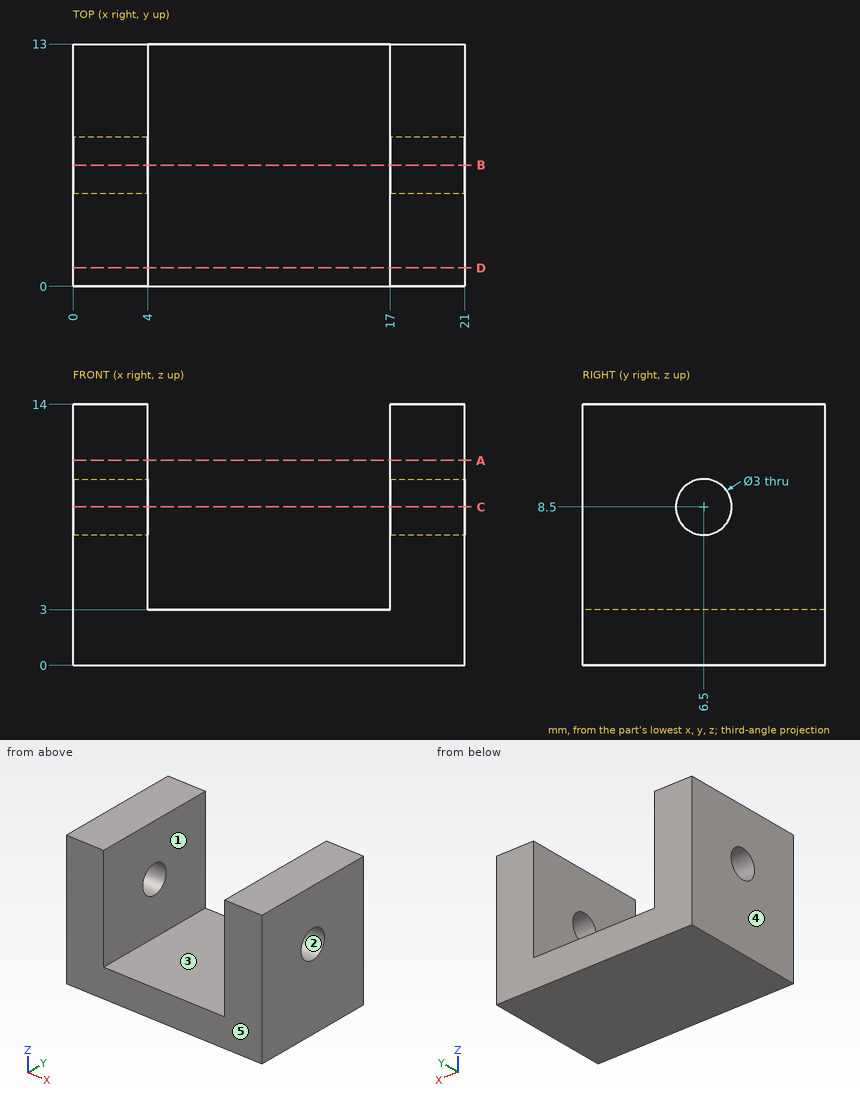
The figure shows three views and two pictorial views of one solid part (mm, origin at its lowest corner). Answer the questions. A direction names the side the tool comes from. Round coordinates to 2 decimals unless told otherwise and drop trailing zeros. Write each loop counter-clockwise with the first axis right and the second up, starting at its lowest first coordinate (ties: lowest second). Pieces come first, ordered by that corner, then holes. Notation, with made-up numbers: (-37.5, 5.25) - (-6.5, 5.25) arc R19 ccw to (-6.5, 11.25) - close; hole circle Ø10 at (85.25, -13.75). An arc over 180 degrees is marked (long way). Use one line per item in the form item = value. Start each with the question number.
Item 1: A cutting plane is placed at A-A (z = 11). Write down the section's boundary in (x, y), plus the area to 3 significant figures.
Item 2: A cutting plane is placed at D-D (y = 1). Write down the section's boundary in (x, z).
Item 3: Determine the mould class of the marked faces 3, 4 and 5 for opening direction X: +X half, -X half, draft (parallel to the pull), parting line (faces both ways), or undercut.
Item 4: A cutting plane is placed at B-B (y = 6.5). Write down the section's boundary in (x, z).
Item 5: Find the intervals of material crossed by line 1 (X direction, y = 3.75, z = 11); line 2 (Z direction, x = 19.9, y = 6.5); line 3 (Z direction, x = 12.5, y = 10.5), in increasing order. Write a range as [from, to].
Item 6: Flat-ended cylindrical pins translate along their axes: pin 1 Ø1.5 at (x, y) = (11, 10.5) entering from +Z; pin 2 Ø4 at (x, z) = (14, 6) entering from -Y. Find the tip coordinate at first contact, or state that the pin passes through.
Item 7: A cutting plane is placed at C-C (z = 8.5). Write down the section's boundary in (x, y).
Item 8: A tool of negligible diameter and unlimited length cuts with its end or side. For the marked faces 1 and 2, from which of +Z, -Z, +X, -X, +Y, -Y can it reach the whole face along a straight path? Write none if from no direction.
The answers:
q1.outline = (0, 0) - (4, 0) - (4, 13) - (0, 13) - close; (17, 0) - (21, 0) - (21, 13) - (17, 13) - close
q1.area = 104 mm^2
q2.outline = (0, 0) - (21, 0) - (21, 14) - (17, 14) - (17, 3) - (4, 3) - (4, 14) - (0, 14) - close
q3.face_3 = undercut
q3.face_4 = -X half
q3.face_5 = draft
q4.outline = (0, 0) - (21, 0) - (21, 7) - (17, 7) - (17, 3) - (4, 3) - (4, 7) - (0, 7) - close; (0, 10) - (4, 10) - (4, 14) - (0, 14) - close; (17, 10) - (21, 10) - (21, 14) - (17, 14) - close
q5.line_1 = [0, 4], [17, 21]
q5.line_2 = [0, 7], [10, 14]
q5.line_3 = [0, 3]
q6.pin_1 = 3
q6.pin_2 = through
q7.outline = (0, 0) - (4, 0) - (4, 5) - (0, 5) - close; (0, 8) - (4, 8) - (4, 13) - (0, 13) - close; (17, 0) - (21, 0) - (21, 5) - (17, 5) - close; (17, 8) - (21, 8) - (21, 13) - (17, 13) - close
q8.face_1 = +Z, +Y, -Y
q8.face_2 = +X, -X
